For this review, take the finished solid that the model builds, in its own axes (mm). A direction names the side the tool comes from. Round coordinates to 2 decimals unless told otherwise and drop trailing zeros. Write each loop counter-clockwise with the first axis right and the second up, starting at its lowest first coordinate (ties: lowest second). Pieces come first, ordered by that corner, then holes. Notation, with made-up numbers: (-23, 49.25) -> (-3, 49.25) arc R36 ccw to (-3, 88.25) -> close; hole circle Ø10 at (2.25, -2). An arc over 180 degrees is marked (long way). Answer as CSV lines item,"result". Start each with the question number.
Item 1: For pin 1 Ø5 at (x, y) = (1, 68.5) entering from +Z; pin 2 Ø20 at (y, z) = (67.5, 51.5) entering from -X; pin 3 Ø1 at (y, z) = (-1, 51.5) entering from -X, all flat-tipped, find the tip position at first contact; note any pin that passes through.
Item 2: Take a section at D-D on x = -14.5. Give the boundary of the cut face in (y, z), then the cut area to 3 significant figures.
Item 3: Mouldability with a two-part tool opening along Y and no side actions: class faces 1 (the flat face through (0, 70, 141.239)), 2 (the flat face through (0, 76.2, 51)), 3 (the cylindrical face through (0.69, 72.95, 115.48)) as +Y half, -Y half, draft (parallel to the pull), parting line (faces both ways), or undercut.
Item 4: Take a section at A-A on x = 0. Give the boundary of the cut face in (y, z) (3 decimals).
Item 5: Machinability: for faces 4 (the flat face through (-25.4, 67, 52)), 5 (the flat face through (-1, 1, 0)), 6 (the flat face through (25.4, 67, 52)), which of the approach directions +Z, -Z, +X, -X, +Y, -Y give a long, thin tool a straight path to every point of the face, cutting with its end or side? Answer none if there is none.
Item 6: Take a section at C-C on z = 85.5. Give the boundary of the cut face in (x, y).
Item 7: Wall thickness on probe 1 along Y at (x, z) = (0.5, 156); probe 2 along X at (y, z) = (-32.5, 25); probe 3 along Y at (x, z) = (23.5, 150): over which ranges is each line inside the solid? List them lowest first. Write a range as from..to.
Item 8: Take a section at B-B on y = 69.85. Give the boundary of the cut face in (x, z) (3 decimals), then the cut area to 3 significant figures.
```python
from build123d import *

# Parameters (mm, degrees)
SKETCH7_R           = 63.5
BOSS_EXTRUDE4_DEPTH = 196.85
SKETCH9_W           = 50.8
SKETCH9_H           = 77.739224187
BOSS_EXTRUDE5_DEPTH = 25.4
SKETCH10_R          = 3.175
BOSS_EXTRUDE6_DEPTH = 50.8


with BuildPart() as part:
    # Sketch7 → Boss-Extrude4 (new body)
    with BuildSketch(Plane.XY):
        Circle(SKETCH7_R)
    extrude(amount=BOSS_EXTRUDE4_DEPTH)

    # Sketch9 → Boss-Extrude5 (add)
    with BuildSketch(Plane(origin=(0, 50.8, 0), x_dir=(1, 0, 0), z_dir=(0, 1, 0))):
        with Locations((0, -51.569612094)):
            Rectangle(SKETCH9_W, SKETCH9_H)
    extrude(amount=BOSS_EXTRUDE5_DEPTH)

    # Sketch10 → Boss-Extrude6 (add)
    with BuildSketch(Plane.XY.offset(90.439224187)):
        with Locations(Location((0, 69.85, 0), (0, 0, 180))):
            Circle(SKETCH10_R)
    extrude(amount=BOSS_EXTRUDE6_DEPTH)


solid = part.part
```
Output values:
1,pin 1,"stops at z = 141.24"
1,pin 2,"stops at x = -26.94"
1,pin 3,"stops at x = -63.5"
2,outline,"(-61.82, 0) -> (61.82, 0) -> (61.82, 12.7) -> (76.2, 12.7) -> (76.2, 90.44) -> (61.82, 90.44) -> (61.82, 196.85) -> (-61.82, 196.85) -> close"
2,area,"25,500 mm^2"
3,face 1,"draft"
3,face 2,"+Y half"
3,face 3,"undercut"
4,outline,"(-63.5, 0) -> (63.5, 0) -> (63.5, 12.7) -> (76.2, 12.7) -> (76.2, 90.439) -> (73.025, 90.439) -> (73.025, 141.239) -> (66.675, 141.239) -> (66.675, 90.439) -> (63.5, 90.439) -> (63.5, 196.85) -> (-63.5, 196.85) -> close"
5,face 4,"+Z, -Z, -X, +Y"
5,face 5,"-Z, +X, -X, +Y, -Y"
5,face 6,"+Z, -Z, +X, +Y"
6,outline,"(-25.4, 58.2) arc R63.5 ccw (long way) to (25.4, 58.2) -> (25.4, 76.2) -> (-25.4, 76.2) -> close"
7,probe 1,"y = -63.5..63.5"
7,probe 2,"x = -54.55..54.55"
7,probe 3,"y = -58.99..58.99"
8,outline,"(-25.4, 12.7) -> (25.4, 12.7) -> (25.4, 90.439) -> (3.175, 90.439) -> (3.175, 141.239) -> (-3.175, 141.239) -> (-3.175, 90.439) -> (-25.4, 90.439) -> close"
8,area,"4,270 mm^2"
